Design review of the part built by this model. Coordinates are the model's own, in mm. Round coordinates to 2 decimals unless told otherwise and drop trailing zeros. Order: outer loops, then holes, each group sorted by start corner. A loop starts at its lowest first (then second) coordinate and runs counter-clockwise, first axis right, second up. Notation, with made-up numbers: (-13, 62) - (31, 62) arc R26 cw to (31, 92) - close; hole circle Ø7 at (36.25, -32). An arc over 180 degrees is marked (long way). Write item = value, one per line.
Autodesk Inventor part; units mm, degrees
ref_plane "YZ Plane" through (0, 0, 0) normal (1, 0, 0) x (0, 1, 0)
ref_plane "XZ Plane" through (0, 0, 0) normal (0, 1, 0) x (-1, 0, 0)
ref_plane "XY Plane" through (0, 0, 0) normal (0, 0, 1) x (1, 0, 0)
sketch "Sketch1" plane through (0, 0, 0) normal (0, 0, 1) x (1, 0, 0)
  circle A0 centre (0, 0) radius 3.2004
  line L0 (0, 0) -> (0, 2.0828)
  line L1 (0, 0) -> (2.0828, 0)
  line L2 (0, 0) -> (0, -2.0828)
  line L3 (0, 0) -> (-2.0828, 0)
  circle A1 centre (0, 2.0828) radius 0.5461
  circle A2 centre (2.0828, 0) radius 0.5461
  circle A3 centre (0, -2.0828) radius 0.5461
  circle A4 centre (-2.0828, 0) radius 0.5461
  dimension "d1" = 2.0828
  dimension "d2" = 2.0828
  dimension "d3" = 2.0828
  dimension "d4" = 2.0828
  dimension "d5" = 1.0922
  dimension "d6" = 1.0922
  dimension "d7" = 1.0922
  dimension "d8" = 1.0922
extrude "Extrusion1" add sketch "Sketch1" along normal blind 0.508
properties part number "cap"
1) Clearance check with a flat-ended pin moving along its axis: pin 1 Ø1 at (x, y) = (2.08, 0) entering from -Z. State where the tip first meets the part, or that it passes through.
Findings:
pin_1 = through
2) We need section C-C on x = -1.75. Write out the cut boundary in (y, z).
Findings:
outline = (-2.68, 0) - (-0.43, 0) - (-0.43, 0.51) - (-2.68, 0.51) - close; (0.43, 0) - (2.68, 0) - (2.68, 0.51) - (0.43, 0.51) - close
3) We need section A-A on y = 0. Write out the cut boundary in (x, z).
Findings:
outline = (-3.2, 0) - (-2.63, 0) - (-2.63, 0.51) - (-3.2, 0.51) - close; (-1.54, 0) - (1.54, 0) - (1.54, 0.51) - (-1.54, 0.51) - close; (2.63, 0) - (3.2, 0) - (3.2, 0.51) - (2.63, 0.51) - close
4) We need section D-D on y = -2.5. Write out the cut boundary in (x, z).
Findings:
outline = (-2, 0) - (-0.35, 0) - (-0.35, 0.51) - (-2, 0.51) - close; (0.35, 0) - (2, 0) - (2, 0.51) - (0.35, 0.51) - close
5) To check wall thickness, follow L1, parallel to Y at x = 0, z = 0.1; L2, parallel to X at y = -0.25, z = 0.1. State the ranges of each line that lie inside material, in increasing order. Write a range as from..to.
Findings:
L1 = -3.2..-2.63, -1.54..1.54, 2.63..3.2
L2 = -3.19..-2.57, -1.6..1.6, 2.57..3.19
6) The part is to be moulded in two halves that separate along X. For faces 1 (the flat face through (0, 0, 0)), 2 (the cylindrical face through (-2.54, 1.95, 0.25)), 3 (the cylindrical face through (-2.63, -0.02, 0.25)), say which applies: released by +X, released by -X, zero draft, split by the parting line, or undercut.
Findings:
face_1 = zero draft
face_2 = split by the parting line
face_3 = undercut
